```python
from build123d import *

# Parameters (mm, degrees)
F0_R     = 9.5
F1_DEPTH = 65
F2_R     = 9.198154
F3_R     = 5.518892
F4_R     = 3.951645
F5_DEPTH = 7


with BuildPart() as f1:
    # F0 (on Right) → F1 (new body)
    with BuildSketch(Plane.YZ):
        Circle(F0_R)
    extrude(amount=F1_DEPTH)

    # F2
    f2_edges = [f1.edges().sort_by_distance(p)[0] for p in [
        (0, -9.5, 0),
    ]]
    fillet(f2_edges, radius=F2_R)

    # F3
    f3_edges = [f1.edges().sort_by_distance(p)[0] for p in [
        (65, -9.5, 0),
    ]]
    fillet(f3_edges, radius=F3_R)

    # F4 (on face) → F5 (join)
    with BuildSketch(Plane.YZ.offset(65)):
        Circle(F4_R)
    extrude(amount=F5_DEPTH)


solid = f1.part
```
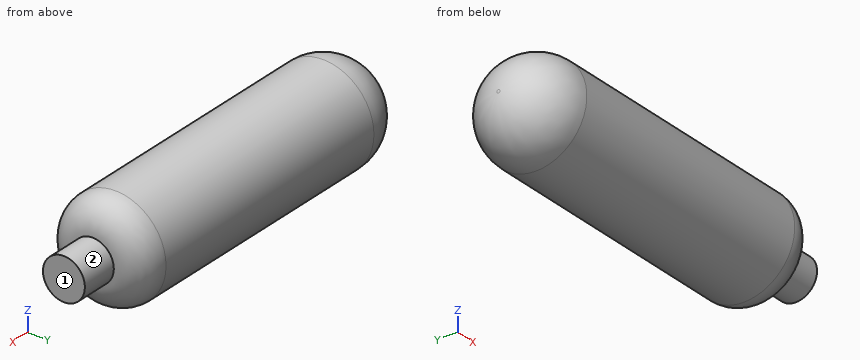
Could you check a few things on this model? Use its own coordinates, in mm. Face numbers are marked on the shaded views. A direction names the side the tool comes from. Coordinates: 2 decimals unless noted, no trailing zeros. Write each loop counter-clockwise with the first axis right and the second up, starting at its lowest first coordinate (ties: lowest second). Pieces come first, ordered by that corner, then holes. Notation, with made-up numbers: (-24, -1) -> (22, -1) arc R34 ccw to (22, 31) -> close; hole circle Ø6 at (60.5, 70). An arc over 180 degrees is marked (long way). Write item = value, one per line. Start each with the question number.
(1) I need wall thicknesses on line 1 (Y direction, x = 16, z = -0.5); line 2 (X direction, y = 2.5, z = -0.75). Which ranges of each line are inside material? Lowest first, please. Write a range as [from, to].
(2) Will these pins go through, and if not, where does the flat tip stop? pin 1 (1 mm diameter, centred on y = -4, z = 2.5, fed in from +X); pin 2 (1.5 mm diameter, centred on x = 33, y = 1, fed in from -Z); pin 3 (3 mm diameter, centred on x = 46, y = 7, fed in from -Z).
(3) I want a section at A-A (x = 11). Please give me the cut outline in (y, z).
(4) Which directions (+Z, -Z, +X, -X, +Y, -Y) give clear straight access to the entire face, cutting with the end or side of a thin tool? Please do the marked faces 1 and 2.
Result set:
q1.line_1 = [-9.49, 9.49]
q1.line_2 = [0.29, 72]
q2.pin_1 = 64.99
q2.pin_2 = -9.5
q2.pin_3 = -7.75
q3.outline = circle Ø19 at (0, 0)
q4.face_1 = +Z, -Z, +X, +Y, -Y
q4.face_2 = +X
